Part model, mm, in its own coordinate system. A direction names the side the tool comes from. Round coordinates to 2 decimals unless told otherwise and drop trailing zeros. Write each loop counter-clockwise with the first axis right and the second up, starting at its lowest first coordinate (ties: lowest second). Pieces come first, ordered by that corner, then holes. Notation, with made-up numbers: M 22,-38.5 L 51,-38.5 A25 cw 51,-17.5 Z; hole C 7.5,-37 d10. An arc over 180 degrees is marked long. Use a Markdown table: item, result. Add a question column.
1) Slice it at B-B on z = 0. Write the cut outline in (x, y), plus the area to 3 significant figures.
2) Wall check: probe 1 along Z at (x, y) = (0, 17.5); probe 2 along Z at (x, y) = (-2, 24.5); probe 3 along X at (y, z) = (5, -4). Give the ranges that are in metal, low to high.
3) Slice it at D-D on x = 3. Write the cut outline in (y, z).
4) Slice it at C-C on y = 36. Write the cut outline in (x, z).
5) Slice it at A-A on x = 0. Write the cut outline in (y, z), plus the area to 3 significant figures.
6) Which spindle directions (+Z, -Z, +X, -X, +Y, -Y) get a long thin tool onto all of the face, cutting with end or side? Do faces 5 (the face through (0, 30, -11)), 6 (the face through (0, 30, 11)), 7 (the face through (0.55, 19.72, -12.488)). Say none if no direction does.
7) Two-plate mould, pull along Z, no slides. Class faces 1 (the face through (-2.4, 19.7, 4.5)), 2 (the face through (0, 35, 10.5)), 3 (the face through (-5.4, 0, -0.2)), 4 (the face through (0, 35, -10.5)): released by +Z, released by -Z, zero draft, split by the parting line, or undercut.
8) Drop flat-ended pins along their axis: P1, Ø10, axis at x = 8, y = 26.5, coming from the -Z side; P2, Ø2, axis at x = 5, y = 12, coming from the +Z side; P3, Ø1, axis at x = -1, z = 12, coming from the +Y side. Give the stop position or say it passes through.
```python
from build123d import *

# Parameters (mm, degrees)
SKETCH_1_R          = 12.5
EXTRUDE_1_DEPTH     = 40
SKETCH_2_W          = 36
SKETCH_2_H          = 27
SKETCH_2_W_2        = 30
SKETCH_2_H_2        = 21
CUT_EXTRUDE_1_DEPTH = 10
HOLE_WIZARD_M12_1_D = 10.2


with BuildPart() as part:
    # 草图1 → 凸台-拉伸1 (new body)
    with BuildSketch(Plane(origin=(0, 0, 0), x_dir=(1, 0, 0), z_dir=(0, 1, 0))):
        with Locations(Location((0, 0, 0), (0, 0, 270))):
            Circle(SKETCH_1_R)
    extrude(amount=EXTRUDE_1_DEPTH)

    # 草图2 → 切除-拉伸1 (cut)
    with BuildSketch(Plane(origin=(0, 40, 0), x_dir=(1, 0, 0), z_dir=(0, 1, 0))):
        Rectangle(SKETCH_2_W, SKETCH_2_H)
        Rectangle(SKETCH_2_W_2, SKETCH_2_H_2, mode=Mode.SUBTRACT)
    extrude(amount=-CUT_EXTRUDE_1_DEPTH, mode=Mode.SUBTRACT)

    # M12 螺纹孔1 (through all)
    with Locations(Plane(origin=(0, 40, 0), x_dir=(1, 0, 0), z_dir=(0, 1, 0))):
        with Locations((0, 0)):
            Hole(HOLE_WIZARD_M12_1_D / 2)


solid = part.part
```
Entries:
| question | item | result |
|---|---|---|
| 1 | outline | M -12.5,0 L -5.1,0 L -5.1,40 L -12.5,40 Z; M 5.1,0 L 12.5,0 L 12.5,40 L 5.1,40 Z |
| 1 | area | 592 mm^2 |
| 2 | probe 1 | z = -12.5 to -5.1, 5.1 to 12.5 |
| 2 | probe 2 | z = -12.34 to -4.69, 4.69 to 12.34 |
| 2 | probe 3 | x = -11.84 to -3.16, 3.16 to 11.84 |
| 3 | outline | M 0,-12.13 L 30,-12.13 L 30,-10.5 L 40,-10.5 L 40,-4.12 L 0,-4.12 Z; M 0,4.12 L 40,4.12 L 40,10.5 L 30,10.5 L 30,12.13 L 0,12.13 Z |
| 4 | outline | M -6.78,-10.5 L 6.78,-10.5 A12.5 ccw 6.78,10.5 L -6.78,10.5 A12.5 ccw Z; hole C 0,0 d10.2 |
| 5 | outline | M 0,-12.5 L 30,-12.5 L 30,-10.5 L 40,-10.5 L 40,-5.1 L 0,-5.1 Z; M 0,5.1 L 40,5.1 L 40,10.5 L 30,10.5 L 30,12.5 L 0,12.5 Z |
| 5 | area | 552 mm^2 |
| 6 | face 5 | -Z, +X, -X, +Y |
| 6 | face 6 | +Z, +X, -X, +Y |
| 6 | face 7 | +Y, -Y |
| 7 | face 1 | undercut |
| 7 | face 2 | released by +Z |
| 7 | face 3 | zero draft |
| 7 | face 4 | released by -Z |
| 8 | P1 | stops at z = -12.13 |
| 8 | P2 | stops at z = 11.84 |
| 8 | P3 | stops at y = 30 |
